Source: three-view drawing plus pictorial views. Frame: mm from the lowest corner of the part. Give positions to 0.01 mm unless a question says otherwise; leave off trailing zeros. Order: outer loops, then holes, each group sorted by start corner. A loop starts at its lowest first (then second) coordinate and runs counter-clockwise, first axis right, second up.
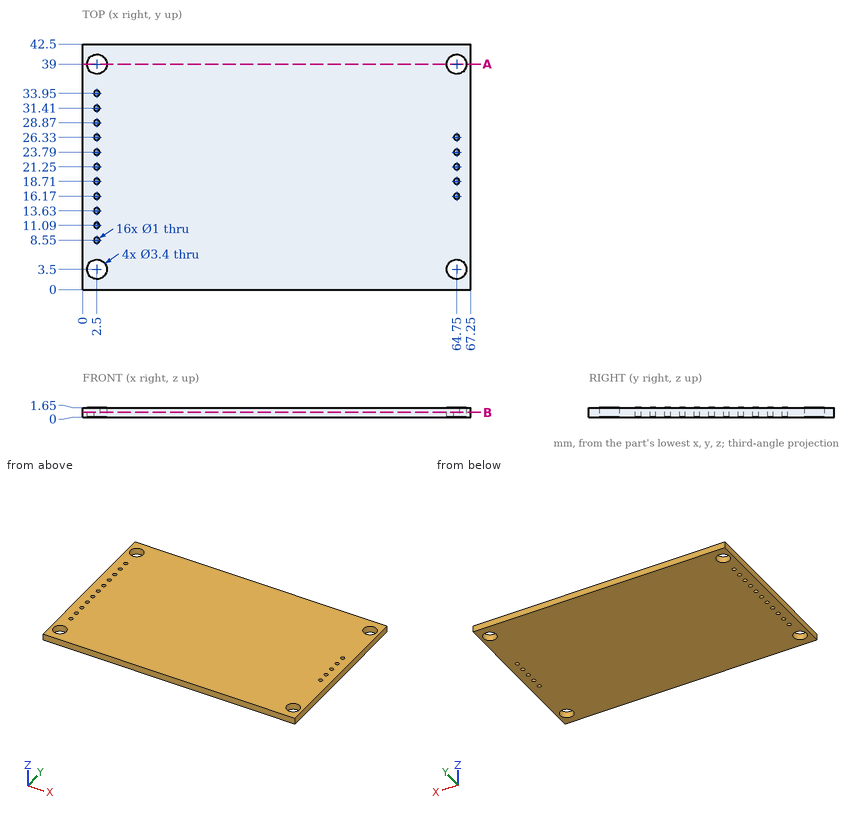
1) Section query B-B on z = 0.8. State how many separate pieces and enclosed holes the cut face has, and give its area (3 significant figures).
Checks:
separate pieces: 1
enclosed holes: 20
area: 2,810 mm2
2) Ray query, L1, parallel to X at y = 34, z = 0.8; L2, parallel to X at y = 5, z = 1; L3, parallel to X at y = 31, z = 1.25. Return the intervals inside material, ascending.
Checks:
L1: x = 0 to 2, 3 to 67.25
L2: x = 0 to 1.7, 3.3 to 63.95, 65.55 to 67.25
L3: x = 0 to 2.21, 2.79 to 67.25
3) Section query A-A on y = 39. Output: boundary loops of the cut face in (x, z), and give its area (3 significant figures).
Checks:
outline: (0, 0) - (0.8, 0) - (0.8, 1.65) - (0, 1.65) - close; (4.2, 0) - (63.05, 0) - (63.05, 1.65) - (4.2, 1.65) - close; (66.45, 0) - (67.25, 0) - (67.25, 1.65) - (66.45, 1.65) - close
area: 99.7 mm2
4) First-contact query: pin 1 Ø2.5 at (x, y) = (64.75, 3.5) entering from -Z. Flat tip, straight axial feed; report the tip coordinate or a pass-through.
Checks:
pin 1: passes through
